For this review, take the finished solid that the model builds, in its own axes (mm). Face numbers are marked on the shaded views. A direction names the side the tool comes from. Coordinates: 2 decimals unless noted, no trailing zeros. Write each loop counter-clockwise with the first axis right and the second up, starting at its lowest first coordinate (ties: lowest second). Pieces come first, ordered by that corner, then holes.
```python
from build123d import *

# Parameters (mm, degrees)
SKETCH1_R                          = 20.6375
BOSS_EXTRUDE1_DEPTH                = 4.7625
SKETCH2_R                          = 8.5328125
BOSS_EXTRUDE2_DEPTH                = 7.9375
F_5_16_0_3125_DIAMETER_HOLE1_D     = 7.9375
F_5_16_0_3125_DIAMETER_HOLE1_DEPTH = 70.104
F_5_16_0_3125_DIAMETER_HOLE1_TIP   = 2.384665582


with BuildPart() as part:
    # Sketch1 → Boss-Extrude1 (new body)
    with BuildSketch(Plane(origin=(0, 0, 0), x_dir=(0, 0, -1), z_dir=(1, 0, 0))):
        with Locations(Location((0, 0, 0), (0, 0, 180))):
            Circle(SKETCH1_R)
    extrude(amount=BOSS_EXTRUDE1_DEPTH)

    # Sketch2 → Boss-Extrude2 (add)
    with BuildSketch(Plane(origin=(4.7625, 0, 0), x_dir=(0, 0, -1), z_dir=(1, 0, 0))):
        Circle(SKETCH2_R)
    extrude(amount=BOSS_EXTRUDE2_DEPTH)

    # 5/16 (0.3125) Diameter Hole1
    with Locations(Plane(origin=(12.7, 0, 0), x_dir=(0, 0, -1), z_dir=(1, 0, 0))):
        with Locations((0, 0)):
            Hole(F_5_16_0_3125_DIAMETER_HOLE1_D / 2, depth=F_5_16_0_3125_DIAMETER_HOLE1_DEPTH)
            with Locations((0, 0, -(F_5_16_0_3125_DIAMETER_HOLE1_DEPTH + F_5_16_0_3125_DIAMETER_HOLE1_TIP / 2))):  # 118° drill point
                Cone(0, F_5_16_0_3125_DIAMETER_HOLE1_D / 2, F_5_16_0_3125_DIAMETER_HOLE1_TIP, mode=Mode.SUBTRACT)


solid = part.part
```
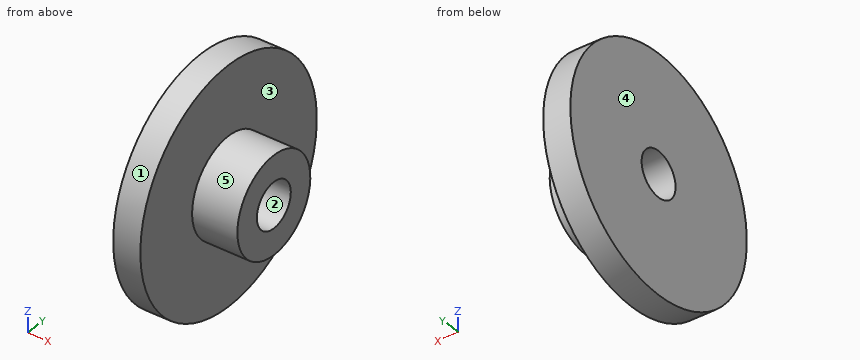
Q1. Add section C-C (x = 2.25). State the section outline as (y, z) points (1 decimal).
Ans:
outline: circle Ø41.3 at (0, 0); hole circle Ø7.9 at (0, 0)
Q2. Tool access review of the marked faces 4 and 5: name each direction out of +Z, -Z, +X, -X, +Y, -Y from which nothing blocks a thin tool from reaching the whole face with its end or side.
Ans:
face 4: +Z, -Z, -X, +Y, -Y
face 5: +X
Q3. For probe 1 along Y at (x, z) = (10, 0); probe 2 along X at (y, z) = (18, 5.5); probe 3 along Y at (x, z) = (0.75, 3.5), list the stretches that pass through material, from the lowest coordinate up.
Ans:
probe 1: y = -8.53 to -3.97, 3.97 to 8.53
probe 2: x = 0 to 4.76
probe 3: y = -20.34 to -1.87, 1.87 to 20.34
Q4. Add section D-D (y = 18.5). State the section outline as (x, z) points, then the cut area to 3 significant figures.
Ans:
outline: (0, -9.15) - (4.76, -9.15) - (4.76, 9.15) - (0, 9.15) - close
area: 87.1 mm2
Q5. Add section A-A (y = 0). State the section outline as (x, z) points.
Ans:
outline: (0, -20.64) - (4.76, -20.64) - (4.76, -8.53) - (12.7, -8.53) - (12.7, -3.97) - (0, -3.97) - close; (0, 3.97) - (12.7, 3.97) - (12.7, 8.53) - (4.76, 8.53) - (4.76, 20.64) - (0, 20.64) - close
Q6. Draft analysis for pull direction Y (two halves, no side actions). For the marked faces 1, 2 and 3, state which applies: +Y half, -Y half, draft (parallel to the pull), parting line (faces both ways), or undercut.
Ans:
face 1: parting line
face 2: undercut
face 3: draft
Q7. Clearance check with flat-ended pins moving along their axes: pin 1 Ø5 at (x, y) = (6, -14) entering from +Z; pin 2 Ø10 at (y, z) = (13.5, 8) entering from +X; pin 3 Ø1 at (x, y) = (11.5, 9.5) entering from -Z; pin 4 Ø5 at (x, z) = (3.5, 16) entering from -Y. State where each tip first meets the part, or that it passes through.
Ans:
pin 1: stops at z = 16.91
pin 2: stops at x = 4.76
pin 3: passes through
pin 4: stops at y = -15.61
